Verification items for this drawing (mm, ordinates from the low corner). A direction names the side the tool comes from. Round coordinates to 2 decimals unless told otherwise and drop trailing zeros. Order: outer loops, then holes, each group sorted by start corner. A loop starts at its lowest first (then second) coordinate and runs counter-clockwise, first axis right, second up. Notation, with made-up numbers: M -24.75,8.5 L 28.25,8.5 A32 cw 28.25,34.5 Z; hole C 39,18 d3. An arc over 180 degrees is marked long. Use CSV: the item, a comma, the result in double quotes. Start each with the question number.
Q1. Scan lines: line 1 (Y direction, x = 8, z = 1.7); line 2 (Y direction, x = 9, z = 2) (1 decimal); line 3 (X direction, y = 65, z = 9). Record each from-to range of solid material in increasing order.
Q2. Gauge pin test, flat ends, axial feed: pin 1 Ø5 at (x, z) = (18.5, 8.5) entering from +Y; pin 2 Ø7.5 at (y, z) = (51.5, 7) entering from +X; pin 3 Ø4.5 at (x, y) = (63, 8.531) entering from +Z; pin 4 Ø1 at (x, z) = (31, 8.5) entering from -Y. Record the tip position at first contact, or that the pin passes through.
Q3. Set-up check for the marked faces 1, 2 and 3: record each of +Z, -Z, +X, -X, +Y, -Y from which the full face is reachable in a straight line by a thin tool's end or side.
Q4. Sectioned sample at A-A (x = 63). Enter the section's corners in (y, z).
Q5. Sectioned sample at C-C (x = 11). Enter the section's corners in (y, z), and give its area (3 significant figures).
Q6. Sectioned sample at D-D (y = 35). Enter the section's corners in (x, z), and give its area (3 significant figures).
Q7. Sectioned sample at B-B (y = 45). Enter the section's corners in (x, z).
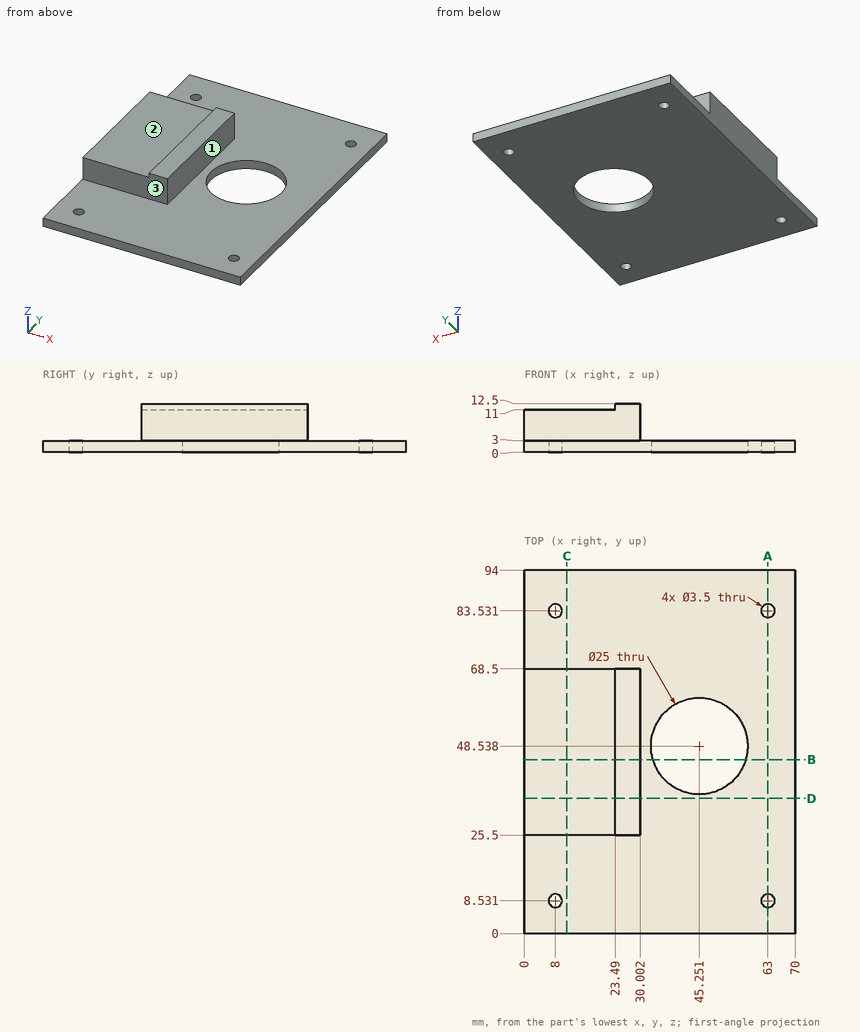
Verdict:
1,line 1,"y = 0 to 6.78, 10.28 to 81.78, 85.28 to 94"
1,line 2,"y = 0 to 7.1, 10 to 82.1, 85 to 94"
1,line 3,"x = 0 to 30"
2,pin 1,"stops at y = 68.5"
2,pin 2,"stops at x = 30"
2,pin 3,"stops at z = 3"
2,pin 4,"passes through"
3,face 1,"+Z, +X, +Y, -Y"
3,face 2,"+Z, -X, +Y, -Y"
3,face 3,"+Z, +X, -X, -Y"
4,outline,"M 0,0 L 6.78,0 L 6.78,3 L 0,3 Z; M 10.28,0 L 81.78,0 L 81.78,3 L 10.28,3 Z; M 85.28,0 L 94,0 L 94,3 L 85.28,3 Z"
5,outline,"M 0,0 L 94,0 L 94,3 L 68.5,3 L 68.5,11 L 25.5,11 L 25.5,3 L 0,3 Z"
5,area,"626 mm²"
6,outline,"M 0,0 L 70,0 L 70,3 L 30,3 L 30,12.5 L 23.49,12.5 L 23.49,11 L 0,11 Z"
6,area,"460 mm²"
7,outline,"M 0,0 L 33.26,0 L 33.26,3 L 30,3 L 30,12.5 L 23.49,12.5 L 23.49,11 L 0,11 Z; M 57.24,0 L 70,0 L 70,3 L 57.24,3 Z"
